Geometry check sheet. Reference: the model listing, model coordinates, mm. Face numbers are marked on the shaded views. Round coordinates to 2 decimals unless told otherwise and drop trailing zeros. Loops run counter-clockwise (first coordinate to the right, second up) from the corner with the lowest first, then second, coordinate; pieces in that order, holes last. Notation, with made-up numbers: M 16,77 L 73,77 A27 cw 73,99 Z; hole C 7.5,54 d6. An arc over 180 degrees is marked long. Answer in a Markdown table with one row per item. Add a question column.
Autodesk Fusion 360 part; units mm, degrees
sketch "Sketch1" plane through (0, 0, 0) normal (0, 0, 1) x (1, 0, 0)
  line L0 (-22, 15) -> (22, 15)
  line L1 (22, 15) -> (22, -15)
  line L2 (22, -15) -> (-22, -15)
  line L3 (-22, -15) -> (-22, 15)
  line L4 (-22, 15) -> (22, -15) construction
  line L5 (22, 15) -> (-22, -15) construction
  line L6 (24.5, 15) -> (22, 15)
  line L7 (22, 15) -> (22, -15)
  line L8 (22, -15) -> (24.5, -15)
  line L9 (24.5, -15) -> (24.5, 15)
  line L10 (-24.5, -15) -> (-22, -15)
  line L11 (-22, -15) -> (-22, 15)
  line L12 (-22, 15) -> (-24.5, 15)
  line L13 (-24.5, 15) -> (-24.5, -15)
  dimension "d1" = 44
  dimension "d2" = 30
  dimension "d8" = 2.5
  dimension "d9" = 2.5
extrude "Extrude1" add sketch "Sketch1" against normal blind 23 contours L3 L10 L11 L12 L13 | L1 L6 L7 L8 L9 makes body 1 at (24.5, -5, -7.6667) makes body 2 at (-22, -5, -7.6667)
extrude "Extrude2" add sketch "Sketch1" along normal blind 12 bodies 1 2
sketch "Sketch2" plane through (-24.5, 0, 0) normal (-1, 0, 0) x (0, -1, 0)
  line L0 (-15, 12) -> (-15, -23)
  line L1 (-15, -23) -> (15, -23)
  line L2 (15, -23) -> (15, 12)
  line L3 (15, 12) -> (-15, 12)
  circle A0 centre (0, -15) radius 3
  dimension "d10" = 6
extrude "Extrude3" cut sketch "Sketch2" against normal blind 24 contours A0 bodies 1
fillet "Fillet1" radius 14.5 4 edges at (-23.25, -15, -23) (-23.25, 15, -23) (23.25, 15, -23) (23.25, -15, -23) on bodies 1
extrude "Extrude4" cut 1 faces at (-7.3333, 5, 0) along direction (0, 0, 1) blind 9 on bodies 1 bodies 1
extrude "Extrude5" cut 1 faces at (-7.3333, 5, 9) along direction (0, 0, 1) blind 0.5 on bodies 1 bodies 1
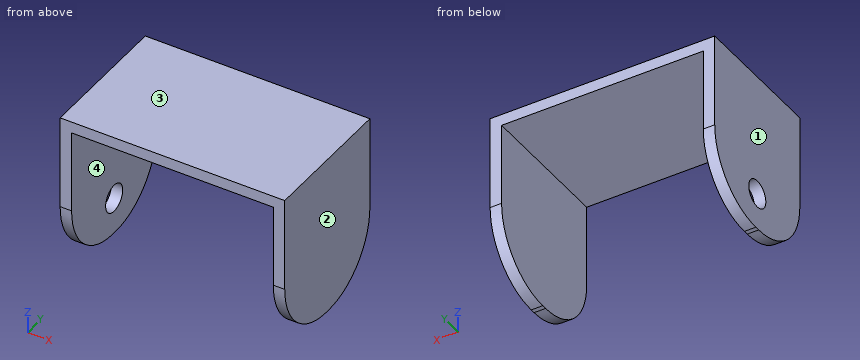
1) Go/stop test with flat-tipped pins: pin 1 (3 mm diameter, centred on x = 19, z = -11.5, fed in from +Y); pin 2 (4 mm diameter, centred on x = 12, y = -1.5, fed in from -Z); pin 3 (1.5 mm diameter, centred on y = 0, z = -16, fed in from -X). Record where each tip stops, or that it passes through.
2) Thickness scan on L1, parallel to Z at x = -24, y = 0; L2, parallel to X at y = -4.5, z = -16; L3, parallel to Z at x = -21, y = 13.5. Record the ranges inside material, lowest first. Write a range as [from, to].
3) Draft check along X on the marked faces 1, 2, 3 and 4. Enter one of: +X half, -X half, draft (parallel to the pull), parting line (faces both ways), or undercut.
4) Cross-section at D-D, the plane y = 2. Record the boundary of the cut face in (x, z).
5) Cross-section at B-B, the plane y = -9. Record the boundary of the cut face in (x, z), plus the area to 3 significant figures.
6) Cross-section at A-A, the plane z = 7. Record the boundary of the cut face in (x, y).
7) Cross-section at C-C, the plane z = -15. Record the boundary of the cut face in (x, y).
Worked answers:
| question | item | result |
|---|---|---|
| 1 | pin 1 | passes through |
| 1 | pin 2 | stops at z = 9.5 |
| 1 | pin 3 | stops at x = 22 |
| 2 | L1 | z = [-23, -18], [-12, 12] |
| 2 | L2 | x = [-24.5, -22], [22, 24.5] |
| 2 | L3 | z = [9.5, 12] |
| 3 | face 1 | -X half |
| 3 | face 2 | +X half |
| 3 | face 3 | draft |
| 3 | face 4 | undercut |
| 4 | outline | M -24.5,-22.92 L -22,-22.92 L -22,-17.24 L -24.5,-17.24 Z; M -24.5,-12.76 L -22,-12.76 L -22,9.5 L 22,9.5 L 22,-22.92 L 24.5,-22.92 L 24.5,12 L -24.5,12 Z |
| 5 | outline | M -24.5,-20.25 L -22,-20.25 L -22,9.5 L 22,9.5 L 22,-20.25 L 24.5,-20.25 L 24.5,12 L -24.5,12 Z |
| 5 | area | 271 mm2 |
| 6 | outline | M -24.5,-15 L -22,-15 L -22,15 L -24.5,15 Z; M 22,-15 L 24.5,-15 L 24.5,15 L 22,15 Z |
| 7 | outline | M -24.5,-13.46 L -22,-13.46 L -22,-3 L -24.5,-3 Z; M -24.5,3 L -22,3 L -22,13.46 L -24.5,13.46 Z; M 22,-13.46 L 24.5,-13.46 L 24.5,13.46 L 22,13.46 Z |
